```python
from build123d import *

# Parameters (mm, degrees)
F0_W     = 144.560187006
F0_H     = 69.128523463
F0_W_2   = 135.035187006
F0_H_2   = 59.603523463
F0_R     = 1.5875
F0_H_3   = 28.9357382685
F0_W_3   = 6.35
F0_H_4   = 127
F1_DEPTH = 3.175
F2_DEPTH = 3.175
F3_DEPTH = 9.525


with BuildPart() as f1:
    # F0 (on Top) → F1 (new body)
    with BuildSketch(Plane.XY):
        Rectangle(F0_W, F0_H)
        Rectangle(F0_W_2, F0_H_2, mode=Mode.SUBTRACT)
        Rectangle(F0_W_2, F0_H_2)
        with Locations((-63.5, -25.4)):
            Circle(F0_R, mode=Mode.SUBTRACT)
        with Locations((63.5, -25.4)):
            Circle(F0_R, mode=Mode.SUBTRACT)
        with Locations((-63.5, 25.4)):
            Circle(F0_R, mode=Mode.SUBTRACT)
        with BuildLine():
            ThreePointArc((63.5, -6.35), (57.9203841816, -19.8203841816), (44.45, -25.4))
            Line((44.45, -25.4), (-44.45, -25.4))
            ThreePointArc((-44.45, -25.4), (-57.9203841816, -19.8203841816), (-63.5, -6.35))
            Line((-63.5, -6.35), (-63.5, 6.35))
            ThreePointArc((-63.5, 6.35), (-57.9203841816, 19.8203841816), (-44.45, 25.4))
            Line((-44.45, 25.4), (44.45, 25.4))
            ThreePointArc((44.45, 25.4), (57.9203841816, 19.8203841816), (63.5, 6.35))
            Line((63.5, 6.35), (63.5, -6.35))
        make_face(mode=Mode.SUBTRACT)
        with Locations((63.5, 25.4)):
            Circle(F0_R, mode=Mode.SUBTRACT)
        Polygon((-120.65, -63.5), (-72.280093503, -63.5), (-72.280093503, -34.5642617315), (-72.280093503, 34.5642617315), (-72.280093503, 63.5), (-120.65, 63.5), align=None)
        with Locations((0, -49.0321308658)):
            Rectangle(F0_W, F0_H_3)
        with Locations((0, 49.0321308658)):
            Rectangle(F0_W, F0_H_3)
        Polygon((72.280093503, -63.5), (101.6, -63.5), (101.6, -9.525), (120.65, 0), (101.6, 9.525), (101.6, 63.5), (72.280093503, 63.5), (72.280093503, 34.5642617315), (72.280093503, -34.5642617315), align=None)
        Polygon((110.612402501, 0), (101.6, -4.5062012505), (101.6, 4.5062012505), align=None, mode=Mode.SUBTRACT)
        with Locations((-123.825, 0)):
            Rectangle(F0_W_3, F0_H_4)
    extrude(amount=F1_DEPTH)

    # F0 (on Top) → F2 (join)
    with BuildSketch(Plane.XY):
        with Locations((0, -49.0321308658)):
            Rectangle(F0_W, F0_H_3)
        Rectangle(F0_W, F0_H)
        Rectangle(F0_W_2, F0_H_2, mode=Mode.SUBTRACT)
        with Locations((0, 49.0321308658)):
            Rectangle(F0_W, F0_H_3)
    extrude(amount=-F2_DEPTH)

    # F0 (on Top) → F3 (join)
    with BuildSketch(Plane.XY):
        with Locations((-123.825, 0)):
            Rectangle(F0_W_3, F0_H_4)
    extrude(amount=-F3_DEPTH)


solid = f1.part
```
Build history of the part. All positions in model axes, mm. A direction names the side the tool comes from. Give positions to 0.01 mm unless a question says otherwise; leave off trailing zeros. Loops run counter-clockwise (first coordinate to the right, second up) from the corner with the lowest first, then second, coordinate; pieces in that order, holes last. Notation, with made-up numbers: (89.25, 53.5) - (100.25, 53.5) arc R34 ccw to (100.25, 86.5) - close; hole circle Ø2 at (-19.5, 53.25). An arc over 180 degrees is marked (long way). Use a Markdown table: item, result.
(1) Which spindle directions (+Z, -Z, +X, -X, +Y, -Y) get a long thin tool onto all of the face, cutting with end or side? Do faces 1 (the face through (-57.77, -19.97, 1.57)), 2 (the face through (-120.65, -1, -5)), 3 (the face through (0, 27, 0)), 4 (the face through (91, 1, 0)). Say none if no direction does.
Taken from the geometry:
| item | result |
|---|---|
| face 1 | +Z, -Z |
| face 2 | -Z, +Y, -Y |
| face 3 | -Z |
| face 4 | -Z, +X, +Y, -Y |
(2) Band-saw the part on B-B (y = -42). Give the cut face in (x, z) (3 decimals), and give its area (3 significant figures).
Taken from the geometry:
| item | result |
|---|---|
| outline | (-127, -9.525) - (-120.65, -9.525) - (-120.65, 0) - (-72.28, 0) - (-72.28, -3.175) - (72.28, -3.175) - (72.28, 0) - (101.6, 0) - (101.6, 3.175) - (-127, 3.175) - close |
| area | 1,250 mm2 |
(3) Wall check: line 1 along X through (y, z) = (-3, -1.5); line 2 along Y through (x, z) = (56, -1); line 3 along X through (y, z) = (1, 1). Give the ranges that are in metal, low to high.
Taken from the geometry:
| item | result |
|---|---|
| line 1 | -127 to -120.65, -72.28 to -67.52, 67.52 to 72.28 |
| line 2 | -63.5 to -29.8, 29.8 to 63.5 |
| line 3 | -127 to -63.5, 63.5 to 101.6, 108.61 to 118.65 |
(4) Band-saw the part on A-A (x = 25.5). Give the cut face in (y, z) (3 decimals), and give its area (3 significant figures).
Taken from the geometry:
| item | result |
|---|---|
| outline | (-63.5, -3.175) - (-29.802, -3.175) - (-29.802, 0) - (-25.4, 0) - (-25.4, 3.175) - (-63.5, 3.175) - close; (25.4, 0) - (29.802, 0) - (29.802, -3.175) - (63.5, -3.175) - (63.5, 3.175) - (25.4, 3.175) - close |
| area | 456 mm2 |
(5) Pull direction X, two halves, no side cores. Call faces 5 (the face through (-127, -1, -3)), 6 (the face through (-58.07, 19.67, 1.57)), 7 (the face through (110.99, -4.83, 1.57)), 8 (the face through (-1, 43, -3.175)): +X half, -X half, draft (parallel to the pull), parting line (faces both ways), or undercut.
Taken from the geometry:
| item | result |
|---|---|
| face 5 | -X half |
| face 6 | undercut |
| face 7 | +X half |
| face 8 | draft |
(6) Band-saw the part on D-D (x = -57). Give the cut face in (y, z) (3 decimals).
Taken from the geometry:
| item | result |
|---|---|
| outline | (-63.5, -3.175) - (-29.802, -3.175) - (-29.802, 0) - (-20.682, 0) - (-20.682, 3.175) - (-63.5, 3.175) - close; (20.682, 0) - (29.802, 0) - (29.802, -3.175) - (63.5, -3.175) - (63.5, 3.175) - (20.682, 3.175) - close |
(7) Drop flat-ended pins along their axis: pin 1 Ø2 at (y, z) = (-22.5, 0) entering from +X; pin 2 Ø1.5 at (y, z) = (19, -5) entering from +X; pin 3 Ø10 at (x, y) = (-95.5, -12.5) entering from -Z. Give the stop position or say it passes through.
Taken from the geometry:
| item | result |
|---|---|
| pin 1 | x = 101.6 |
| pin 2 | x = -120.65 |
| pin 3 | z = 0 |
(8) Band-saw the part on C-C (x = -110). Give the cut face in (y, z) (3 decimals), and give its area (3 significant figures).
Taken from the geometry:
| item | result |
|---|---|
| outline | (-63.5, 0) - (63.5, 0) - (63.5, 3.175) - (-63.5, 3.175) - close |
| area | 403 mm2 |
